CAD build for the part. Positions are in the model's coordinates, mm. A direction names the side the tool comes from. Round coordinates to 2 decimals unless told otherwise and drop trailing zeros. Loops run counter-clockwise (first coordinate to the right, second up) from the corner with the lowest first, then second, coordinate; pieces in that order, holes last.
```python
from build123d import *

# Parameters (mm, degrees)
F4_R      = 2.54
F8_DEPTH  = 450.088
F10_DEPTH = 6.35


with BuildPart() as f2:
    # F2: sweep along a path in F0
    with BuildLine(Plane.XZ) as f2_path:
        Line((203.2, 0), (203.2, 76.2))
        ThreePointArc((203.2, 76.2), (180.8815367264, 130.0815367264), (127, 152.4))
        Line((127, 152.4), (0, 152.4))
    # F1 (on Top) → F2 (sweep)
    with BuildSketch(Plane.XY):
        with BuildLine():
            ThreePointArc((190.5, 0), (203.2, -12.7), (215.9, 0))
            ThreePointArc((215.9, 0), (203.2, 12.7), (190.5, 0))
        make_face()
    sweep(path=f2_path.line)

    # F3: F2 across plane


with BuildPart() as f2_1:
    add(f2.part)
    add(f2.part.mirror(Plane.YZ))

    # F4
    f4_edges = [f2_1.edges().sort_by_distance(p)[0] for p in [
        (190.5, 0, 0),
        (-190.5, 0, 0),
    ]]
    fillet(f4_edges, radius=F4_R)

    # F7 (on offset) → F8 (cut)
    with BuildSketch(Plane.YZ.offset(215.9)):
        with BuildLine():
            ThreePointArc((0, 22.225), (2.2450640303, 23.1549359697), (3.175, 25.4))
            ThreePointArc((3.175, 25.4), (-2.2450640303, 27.6450640303), (0, 22.225))
        make_face()
    extrude(amount=-F8_DEPTH, mode=Mode.SUBTRACT)

    # F9 (on offset) → F10 (cut)
    with BuildSketch(Plane.YZ.offset(-215.9)):
        with BuildLine():
            ThreePointArc((0, 22.225), (2.2450640303, 23.1549359697), (3.175, 25.4))
            ThreePointArc((3.175, 25.4), (-2.2450640303, 27.6450640303), (0, 22.225))
        make_face()
    extrude(amount=F10_DEPTH, mode=Mode.SUBTRACT)


solid = f2_1.part
```
Item 1: Cut at A-A, the plane z = 43. Give the cut face in (x, y).
Answers follow:
outline: circle Ø25.4 at (-203.2, 0); circle Ø25.4 at (203.2, 0)
Item 2: Flat gauge pins, fed straight in: P1, Ø2, axis at y = -9, z = 130, coming from the -X side; P2, Ø8, axis at y = -2.5, z = 90.5, coming from the -X side; P3, Ø1, axis at x = -6, y = 9, coming from the +Z side; P4, Ø10, axis at y = 0, z = 25.4, coming from the +X side. Where does each tip first touch, or does it go through?
Answers follow:
P1: stops at x = -194.44
P2: stops at x = -215.23
P3: stops at z = 161.84
P4: stops at x = 215.9
Item 3: 3-axis set-ups, long thin cutter, end or side, ignore diameter. For faces 3 (the cylindrical face through (214.932, -4.864, 39.886)), 4 (the cylindrical face through (1.778, 0.558, 139.712)), 5 (the flat face through (-203, 0, 0)): which of +Z, -Z, +X, -X, +Y, -Y reach the whole face in a straight line?
Answers follow:
face 3: -Z
face 4: none
face 5: -Z, +X, -X, +Y, -Y
Item 4: Two-plate mould, pull along X, no slides. Class faces 1 (the flat face through (203, 0, 0)), 2 (the cylindrical face through (-214.932, -4.864, 39.886)): released by +X, released by -X, zero draft, split by the parting line, or undercut.
Answers follow:
face 1: zero draft
face 2: undercut
Item 5: Cut at B-B, the plane x = 51. Give the cut face in (y, z), plus the area to 3 significant figures.
Answers follow:
outline: circle Ø25.4 at (0, 152.4)
area: 507 mm2
Item 6: Probe line 1 (Y direction, x = 204.5, z = 25.4) (3 decimals); line 2 (X direction, y = -7.5, z = 62.5); line 3 (Z direction, x = -4, y = -0.5). List the from-to ranges inside material, lowest first.
Answers follow:
line 1: y = -12.633 to -3.175, 3.175 to 12.633
line 2: x = -213.45 to -192.95, 192.95 to 213.45
line 3: z = 139.71 to 165.09
